from build123d import *

# Parameters (mm, degrees)
BOSS_EXTRUDE1_DEPTH                               = 3.175
F_6_CLEARANCE_HOLE1_D                             = 4.3053
SKETCH7_R                                         = 19.84375
SKETCH7_R_2                                       = 6.35
CUT_EXTRUDE1_DEPTH                                = 4.175
CSK_FOR_6_FLAT_HEAD_MACHINE_SCREW_100_D           = 4.3053
CSK_FOR_6_FLAT_HEAD_MACHINE_SCREW_100_DEPTH       = 3.175
CSK_FOR_6_FLAT_HEAD_MACHINE_SCREW_100_CSINK_D     = 7.0866
CSK_FOR_6_FLAT_HEAD_MACHINE_SCREW_100_CSINK_ANGLE = 100


with BuildPart() as part:
    # Sketch1 → Boss-Extrude1 (new body)
    with BuildSketch(Plane.XY):
        Polygon((0, 97.282), (-146.05, 33.02), (-146.05, 0), (0, 0), align=None)
    extrude(amount=-BOSS_EXTRUDE1_DEPTH)

    # #6 Clearance Hole1 (through all)
    with Locations(Plane(origin=(0, 0, -3.175), x_dir=(-1, 0, 0), z_dir=(0, 0, -1))):
        with Locations((4.8895, 80.9625), (4.8895, 14.2875), (141.1605, 14.2875), (11.176, 28.575), (60.325, 46.0375), (99.06, 14.2875)):
            Hole(F_6_CLEARANCE_HOLE1_D / 2)

    # Sketch7 → Cut-Extrude1 (cut, through all)
    with BuildSketch(Plane(origin=(0, 0, -3.175), x_dir=(-1, 0, 0), z_dir=(0, 0, -1))):
        with Locations((32.004, 59.944)):
            Circle(SKETCH7_R)
        with Locations((28.575, 19.375884027)):
            Circle(SKETCH7_R_2)
        with Locations((73.025, 19.558)):
            Circle(SKETCH7_R_2)
        with Locations((117.475, 19.558)):
            Circle(SKETCH7_R_2)
    extrude(amount=-CUT_EXTRUDE1_DEPTH, mode=Mode.SUBTRACT)

    # CSK for #6 Flat Head Machine Screw (100)1
    with Locations(Plane(origin=(0, 0, -3.175), x_dir=(-1, 0, 0), z_dir=(0, 0, -1))):
        with Locations((8.904042987, 61.838331605), (55.103957013, 58.049668395)):
            CounterSinkHole(CSK_FOR_6_FLAT_HEAD_MACHINE_SCREW_100_D / 2, CSK_FOR_6_FLAT_HEAD_MACHINE_SCREW_100_CSINK_D / 2, depth=CSK_FOR_6_FLAT_HEAD_MACHINE_SCREW_100_DEPTH, counter_sink_angle=CSK_FOR_6_FLAT_HEAD_MACHINE_SCREW_100_CSINK_ANGLE)


solid = part.part
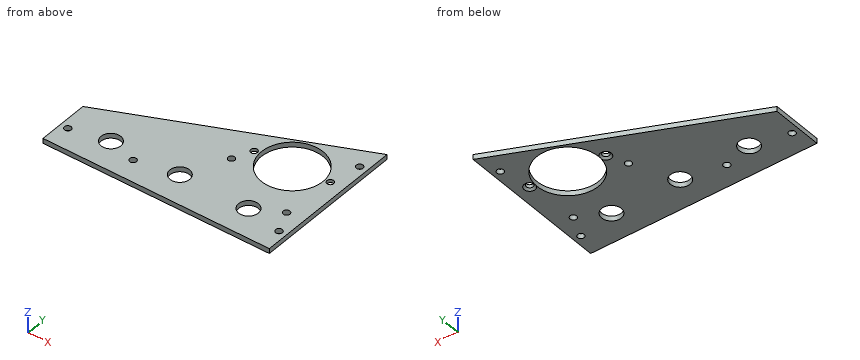
The listing builds one solid part. Answer for the finished solid, in the listing's coordinates (mm). Coordinates: 2 decimals unless noted, no trailing zeros. Order: outer loops, then holes, each group sorted by start corner. A loop starts at its lowest first (then second) coordinate and runs counter-clockwise, first axis right, second up. Notation, with made-up numbers: M 11.25,11.5 L 62.25,11.5 A14 cw 62.25,18.5 Z; hole C 36.5,52 d3. An arc over 180 degrees is marked long. Use CSV: the item, a comma, the result in double quotes.
Q1. Straight lines are drawn through the part: L1, parallel to X at y = 19.5, z = -2.1; L2, parallel to X at y = 24, z = -0.55; L3, parallel to Y at x = -9.5, z = -2.15. For each, find the intervals that lie inside material, in ascending order.
Here are the results:
L1,"-146.05 to -123.82, -111.13 to -79.37, -66.68 to -34.92, -22.23 to 0"
L2,"-146.05 to -122.01, -112.94 to -77.56, -68.49 to -32.93, -24.22 to 0"
L3,"0 to 27.22, 29.93 to 59.59, 64.08 to 93.1"
Q2. Section D-D (x = -133) is taken. Determine the outline of the cut face in (y, z) (3 decimals), then the cut area to 3 significant figures.
Here are the results:
outline,"M 0,-3.175 L 38.762,-3.175 L 38.762,0 L 0,0 Z"
area,"123 mm2"
Q3. Given pin 1 Ø5.5 at (x, y) = (-55.1, 58.05) entering from -Z; pin 2 Ø1 at (y, z) = (74.5, -0.5) entering from +X, each flat-ended and moving along its own axis, determine where each tip first touches the part or whether it passes through.
Here are the results:
pin 1,"z = -2.51"
pin 2,"x = 0"
Q4. Section A-A (x = -16) is taken. Determine the outline of the cut face in (y, z) (3 decimals), then the cut area to 3 significant figures.
Here are the results:
outline,"M 0,-3.175 L 48.212,-3.175 L 48.212,0 L 0,0 Z; M 71.676,-3.175 L 90.242,-3.175 L 90.242,0 L 71.676,0 Z"
area,"212 mm2"
Q5. Section B-B (z = -0.8) is taken. Give the number of separate pieces and of enclosed holes in the cut face, then the cut area to 3 significant figures.
Here are the results:
separate pieces,"1"
enclosed holes,"12"
area,"7,780 mm2"
Q6. Section C-C (x = -99.06) is taken. Determine the outline of the cut face in (y, z) (3 decimals), then the cut area to 3 significant figures.
Here are the results:
outline,"M 0,-3.175 L 12.135,-3.175 L 12.135,0 L 0,0 Z; M 16.44,-3.175 L 53.696,-3.175 L 53.696,0 L 16.44,0 Z"
area,"157 mm2"
